Input: dimensioned drawing with shaded views. Units: mm. Origin: part minimum x, y, z. A direction names the side the tool comes from. Round coordinates to 2 decimals unless told otherwise and drop trailing zeros. Loops run counter-clockwise (first coordinate to the right, second up) from the corner with the lowest first, then second, coordinate; pieces in that order, holes last.
Item 1: Pull-direction query (Y, two-part tool) for the marked faces 6, 7 and 8; classes: released by +Y, released by -Y, zero draft, split by the parting line, or undercut.
Item 2: Section query C-C on x = 6. Return loops of the section in (y, z).
Item 3: Access query for the marked faces 1, 2, 3, 4 and 5. Directions: +Z, -Z, +X, -X, +Y, -Y. A direction counts if a zero-diameter tool reaches every point of the face in a straight line with its end or side. Return the directions, or none.
Item 4: Ray query, L1, parallel to X at y = 30.5, z = 3.25; L2, parallel to X at y = 14, z = 4; L3, parallel to Z at x = 30, y = 16.75. Return the intervals inside material, ascending.
Item 5: Section query B-B on y = 23.5. Return loops of the section in (x, z).
Item 6: Section query A-A on z = 5.5. Return loops of the section in (x, y).
Item 7: Section query D-D on x = 25. Return loops of the section in (y, z), then the cut area to 3 significant figures.
Item 8: First-contact query: P1, Ø1, axis at x = 10.5, z = 5, coming from the -Y side; P2, Ø3.5, axis at y = 4, z = 1.5, coming from the +X side; P3, Ø3, axis at y = 2.5, z = 4.5, coming from the -X side. Flat tips, straight axial feed; report the tip coordinate or a pass-through.
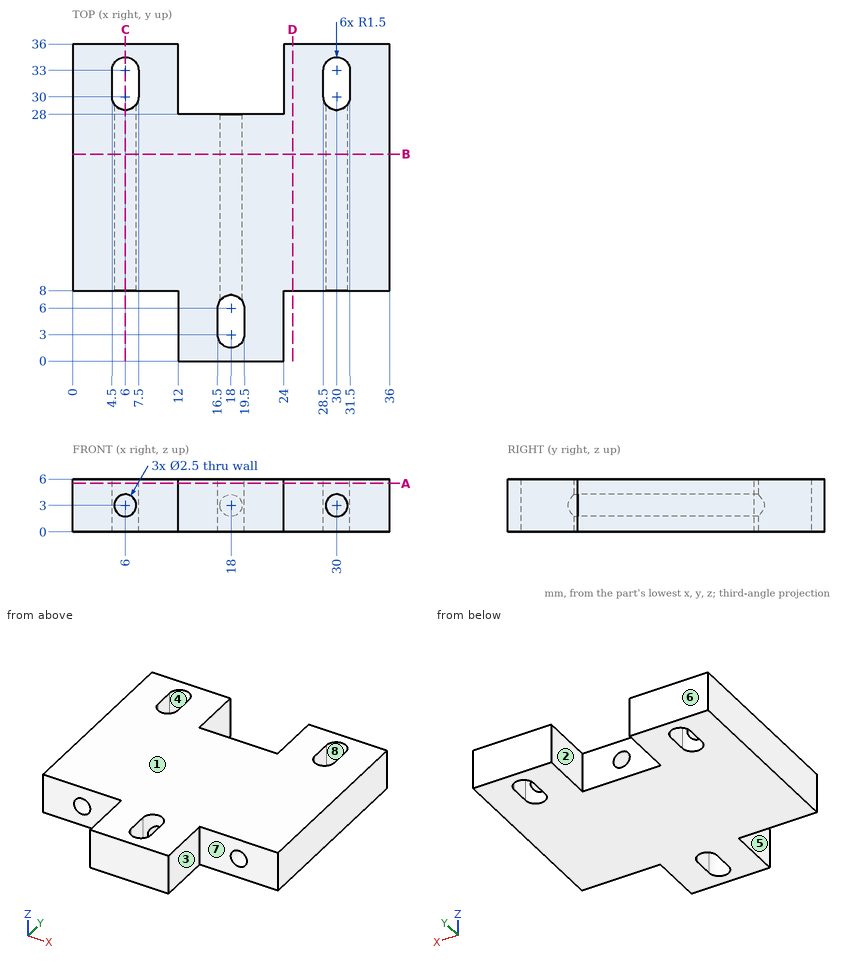
Data:
1. face 6: released by +Y
1. face 7: released by -Y
1. face 8: undercut
2. outline: (8, 0) - (28.5, 0) - (28.5, 1.75) - (8, 1.75) - close; (8, 4.25) - (28.5, 4.25) - (28.5, 6) - (8, 6) - close; (34.5, 0) - (36, 0) - (36, 6) - (34.5, 6) - close
3. face 1: +Z, +X, -X, +Y, -Y
3. face 2: +Z, -Z, +Y
3. face 3: +Z, -Z, +X, -Y
3. face 4: +Z, -Z
3. face 5: +Z, -Z, -X, -Y
4. L1: x = 0 to 4.5, 7.5 to 12, 24 to 28.5, 31.5 to 36
4. L2: x = 0 to 5.25, 6.75 to 17.25, 18.75 to 29.25, 30.75 to 36
4. L3: z = 0 to 1.75, 4.25 to 6
5. outline: (0, 0) - (36, 0) - (36, 6) - (0, 6) - close; hole circle Ø2.5 at (6, 3); hole circle Ø2.5 at (18, 3); hole circle Ø2.5 at (30, 3)
6. outline: (0, 8) - (12, 8) - (12, 0) - (24, 0) - (24, 8) - (36, 8) - (36, 36) - (24, 36) - (24, 28) - (12, 28) - (12, 36) - (0, 36) - close; hole (4.5, 30) arc R1.5 ccw to (7.5, 30) - (7.5, 33) arc R1.5 ccw to (4.5, 33) - close; hole (16.5, 3) arc R1.5 ccw to (19.5, 3) - (19.5, 6) arc R1.5 ccw to (16.5, 6) - close; hole (28.5, 30) arc R1.5 ccw to (31.5, 30) - (31.5, 33) arc R1.5 ccw to (28.5, 33) - close
7. outline: (8, 0) - (36, 0) - (36, 6) - (8, 6) - close
7. area: 168 mm2
8. P1: stops at y = 8
8. P2: stops at x = 24
8. P3: stops at x = 12
